Build history of the part. All positions in model axes, mm. A direction names the side the tool comes from. Round coordinates to 2 decimals unless told otherwise and drop trailing zeros. Write each loop counter-clockwise with the first axis right and the second up, starting at its lowest first coordinate (ties: lowest second). Pieces come first, ordered by that corner, then holes.
Item 1: 3-axis set-ups, long thin cutter, end or side, ignore diameter. For faces 3 (the flat face through (-15, 36, -78)), 4 (the flat face through (-65.25, 12.465, -37.914)), 5 (the cylindrical face through (92.298, 20.706, -0.101)): which of +Z, -Z, +X, -X, +Y, -Y reach the whole face in a straight line?
Item 2: Wall check: probe 1 along Z at (x, y) = (58.5, 31); probe 2 along X at (y, z) = (23.5, 29.5); probe 3 along X at (y, z) = (28, 87.5). Give the ranges that are in metal, low to high.
Item 3: Band-saw the part on B-B, the plane x = -45. Write the cut outline in (y, z).
Item 4: Drop flat-ended pins along their axis: pin 1 Ø1.9 at (x, z) = (-72.55, 30.34) entering from -Y; pin 2 Ø2 at (x, y) = (-71, 27) entering from +Z; pin 3 Ø3 at (y, z) = (37, -79) entering from -X; pin 4 Ø8 at (y, z) = (30, 54) entering from +X. Give the stop position or say it passes through.
Item 5: Band-saw the part on C-C, the plane y = 37. Count the separate pieces of the cut face and the enclosed holes in it, then the cut area to 3 significant figures.
Item 6: Band-saw the part on A-A, the plane z = 0. Write the cut outline in (x, y), then the cut area to 3 significant figures.
Item 7: Mould opens along X. For faces 1 (the cylindrical face through (92.74, 20.71, 20.59)), 2 (the flat face through (-75.111, 36.062, -26.045)) say: +X half, -X half, draft (parallel to the pull), parting line (faces both ways), or undercut.
```python
from build123d import *

# Parameters (mm, degrees)
SKETCH1_R             = 95
SKETCH1_R_2           = 70
BOSS_EXTRUDE1_DEPTH   = 42
CUT_EXTRUDE3_DEPTH    = 15
CIRPATTERN2_COUNT     = 6
M3_CLEARANCE_HOLE1_D  = 3.2
F_5_0MM_DOWEL_SLOT1_D = 4.6


with BuildPart() as part:
    # Sketch1 → Boss-Extrude1 (new body)
    with BuildSketch(Plane(origin=(0, 0, 0), x_dir=(1, 0, 0), z_dir=(0, 1, 0))):
        with Locations(Location((0, 0, 0), (0, 0, 90))):
            Circle(SKETCH1_R)
        with Locations(Location((0, 0, 0), (0, 0, 90))):
            Circle(SKETCH1_R_2, mode=Mode.SUBTRACT)
    extrude(amount=BOSS_EXTRUDE1_DEPTH)

    # Sketch7 → Cut-Extrude3 (cut, symmetric)
    with BuildSketch(Plane(origin=(0, 0, 0), x_dir=(0, -1, 0), z_dir=(-0.500000000000001, 0, 0.866025403784438))):
        Polygon((-42, 83), (-32, 83), (-27, 78), (-32, 73), (-42, 73), align=None)
        Polygon((-10, 83), (0, 83), (0, 73), (-10, 73), (-15, 78), align=None)
    cut_extrude3 = extrude(amount=CUT_EXTRUDE3_DEPTH, both=True, mode=Mode.SUBTRACT)

    # CirPattern2: Cut-Extrude3 ×6 about axis
    cirpattern2_axis = Axis((0, 0, 0), (0, 1, 0))
    for i in range(1, CIRPATTERN2_COUNT):
        add(cut_extrude3.rotate(cirpattern2_axis, i * 360 / CIRPATTERN2_COUNT), mode=Mode.SUBTRACT)

    # M3 Clearance Hole1 (through all)
    with Locations(Plane(origin=(0, 42, 0), x_dir=(1, 0, 0), z_dir=(0, 1, 0))):
        with Locations((62.549981495, -47.660254038), (72.549981495, -30.339745962), (-10, -78), (10, -78), (-72.549981495, -30.339745962), (-62.549981495, -47.660254038), (-62.549981495, 47.660254038), (-72.549981495, 30.339745962), (10, 78), (-10, 78), (72.549981495, 30.339745962), (62.549981495, 47.660254038), (0, 0)):
            Hole(M3_CLEARANCE_HOLE1_D / 2)

    # Ø5.0mm Dowel Slot1 (through all)
    with Locations(Plane(origin=(0, 42, 0), x_dir=(1, 0, 0), z_dir=(0, 1, 0))):
        with Locations((0, 90), (23.293714059, 86.933324366), (45, 77.942286341), (63.639610307, 63.639610307), (77.942286341, 45), (86.933324366, 23.293714059), (90, 0), (86.933324366, -23.293714059), (77.942286341, -45), (63.639610307, -63.639610307), (45, -77.942286341), (23.293714059, -86.933324366), (0, -90), (-23.293714059, -86.933324366), (-45, -77.942286341), (-63.639610307, -63.639610307), (-77.942286341, -45), (-86.933324366, -23.293714059), (-90, 0), (-86.933324366, 23.293714059), (-77.942286341, 45), (-63.639610307, 63.639610307), (-45, 77.942286341), (-23.293714059, 86.933324366), (0, 0)):
            Hole(F_5_0MM_DOWEL_SLOT1_D / 2)


solid = part.part
```
Results:
1. face 3: +Y
1. face 4: -Y
1. face 5: +Y, -Y
2. probe 1: z = -74.85 to -51.1, -46.68 to -38.44, 38.44 to 46.68, 51.1 to 74.85
2. probe 2: x = -90.3 to -73.91, -71.19 to -63.48, 63.48 to 71.19, 73.91 to 90.3
2. probe 3: x = -37 to -25.52, -21.06 to 21.06, 25.52 to 37
3. outline: (0, -83.67) - (42, -83.67) - (42, -80.24) - (0, -80.24) - close; (0, -75.64) - (42, -75.64) - (42, -53.62) - (0, -53.62) - close; (0, 53.62) - (42, 53.62) - (42, 75.64) - (0, 75.64) - close; (0, 80.24) - (42, 80.24) - (42, 83.67) - (0, 83.67) - close
4. pin 1: passes through
4. pin 2: stops at z = 64.23
4. pin 3: stops at x = -54.94
4. pin 4: stops at x = 80.78
5. separate pieces: 1
5. enclosed holes: 31
5. area: 10,800 mm2
6. outline: (-95, 0) - (-92.3, 0) - (-92.3, 42) - (-95, 42) - close; (-87.7, 0) - (-70, 0) - (-70, 42) - (-87.7, 42) - close; (70, 0) - (87.7, 0) - (87.7, 42) - (70, 42) - close; (92.3, 0) - (95, 0) - (95, 42) - (92.3, 42) - close
6. area: 1,710 mm2
7. face 1: parting line
7. face 2: undercut
